Design review of the part built by this model. Coordinates are the model's own, in mm. Face numbers are marked on the shaded views. A direction names the side the tool comes from. Give positions to 0.01 mm unless a question says otherwise; leave off trailing zeros. Write each loop counter-clockwise with the first axis right and the second up, starting at its lowest first coordinate (ties: lowest second). Pieces come first, ordered by that corner, then holes. Notation, with made-up numbers: (5, 60.25) -> (38, 60.25) arc R7 ccw to (38, 72.25) -> close; hole circle Ø11 at (-31.5, 2). An arc over 180 degrees is marked (long way). Return JSON: item names as keys, results as strings. Group by question number.
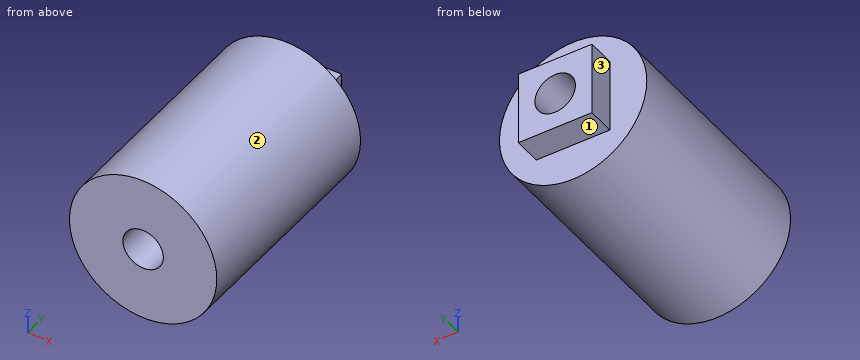
Autodesk Inventor part; units mm, degrees
ref_plane "YZ Plane" through (0, 0, 0) normal (1, 0, 0) x (0, 1, 0)
ref_plane "XZ Plane" through (0, 0, 0) normal (0, 1, 0) x (-1, 0, 0)
ref_plane "XY Plane" through (0, 0, 0) normal (0, 0, 1) x (1, 0, 0)
sketch "Sketch1" plane through (0, 0, 0) normal (0, 1, 0) x (-1, 0, 0)
  circle A0 centre (0, 0) radius 4
  dimension "d0" = 8
extrude "Extrusion1" add sketch "Sketch1" along normal blind 12
sketch "Sketch2" plane through (0, 12, 0) normal (0, 1, 0) x (1, 0, 0)
  line L0 (-2, -2) -> (2, -2)
  line L1 (2, -2) -> (2, 2)
  line L2 (2, 2) -> (-2, 2)
  line L3 (-2, 2) -> (-2, -2)
  point P0 (0, 0)
  dimension "d3" = 4
  dimension "d4" = 4
  dimension "d5" = 2
  dimension "d6" = 2
extrude "Extrusion2" add sketch "Sketch2" along normal blind 1.5
sketch "Sketch3" plane through (0, 13.5, 0) normal (0, 1, 0) x (1, 0, 0)
  circle A0 centre (0, 0) radius 1.1
  dimension "d9" = 2.2
extrude "Extrusion3" cut sketch "Sketch3" against normal through all
properties part number "axe_top"
Q1. Insertion check: pin 1 (4 mm diameter, centred on x = -1, y = 8, fed in from +Z); pin 2 (0.8 mm diameter, centred on y = 12.5, z = 1, fed in from +X); pin 3 (1.2 mm diameter, centred on x = -0.5, y = 13, fed in from +Z). Each pin has a flat end and moves straight along its axis. Give the tip position at first contact, or say it passes through.
Q2. Take a section at B-B, the plane z = 0. Give the boundary of the cut face in (x, y).
Q3. Take a section at D-D, the plane y = 3.25. Give the boundary of the cut face in (x, z), plus the area to 3 significant figures.
Q4. Take a section at C-C, the plane z = -1.25. Give the boundary of the cut face in (x, y), plus the area to 3 significant figures.
Q5. Tool access review of the marked faces 1, 2 and 3: name each direction out of +Z, -Z, +X, -X, +Y, -Y from which nothing blocks a thin tool from reaching the whole face with its end or side.
Q6. Take a section at A-A, the plane x = 0. Give the boundary of the cut face in (y, z), plus the area to 3 significant figures.
Q7. For L1, parallel to Z at x = 0, y = 8.5; L2, parallel to Y at x = 1, z = 2.5; L3, parallel to Z at x = 1, y = 1.75, list the stretches that pass through material, from the lowest coordinate up. Write a range as from..to.
Final values:
{
 "1": {"pin 1": "stops at z = 4", "pin 2": "stops at x = 2", "pin 3": "stops at z = 2"},
 "2": {"outline": "(-4, 0) -> (-1.1, 0) -> (-1.1, 13.5) -> (-2, 13.5) -> (-2, 12) -> (-4, 12) -> close; (1.1, 0) -> (4, 0) -> (4, 12) -> (2, 12) -> (2, 13.5) -> (1.1, 13.5) -> close"},
 "3": {"outline": "circle Ø8 at (0, 0); hole circle Ø2.2 at (0, 0)", "area": "46.5 mm²"},
 "4": {"outline": "(-3.8, 0) -> (3.8, 0) -> (3.8, 12) -> (2, 12) -> (2, 13.5) -> (-2, 13.5) -> (-2, 12) -> (-3.8, 12) -> close", "area": "97.2 mm²"},
 "5": {"face 1": "-Z, +X, -X, +Y", "face 2": "+Y, -Y", "face 3": "+Z, -Z, -X, +Y"},
 "6": {"outline": "(0, -4) -> (12, -4) -> (12, -2) -> (13.5, -2) -> (13.5, -1.1) -> (0, -1.1) -> close; (0, 1.1) -> (13.5, 1.1) -> (13.5, 2) -> (12, 2) -> (12, 4) -> (0, 4) -> close", "area": "72.3 mm²"},
 "7": {"L1": "z = -4..-1.1, 1.1..4", "L2": "y = 0..12", "L3": "z = -3.87..-0.46, 0.46..3.87"}
}
